from build123d import *

# Parameters (mm, degrees)
F1_DEPTH = 774.7
F2_W     = 304.8
F2_H     = 165.1
F2_R     = 15.875
F2_W_2   = 203.2
F3_DEPTH = 25.4
F4_W     = 88.9
F4_H     = 558.8
F4_R     = 14.2875
F5_DEPTH = 38.1
F6_W     = 12.7
F6_H     = 698.5
F7_DEPTH = 406.4


with BuildPart() as f1:
    # F0 (on Right) → F1 (new body, symmetric)
    with BuildSketch(Plane.YZ):
        with BuildLine():
            Line((-488.95, 12.7), (-488.95, 0))
            Line((-488.95, 0), (-381, 0))
            ThreePointArc((-381, 0), (-358.54936, 9.29936), (-349.25, 31.75))
            Line((-349.25, 31.75), (-349.25, 387.35))
            ThreePointArc((-349.25, 387.35), (-343.670384, 400.820384), (-330.2, 406.4))
            Line((-330.2, 406.4), (0, 406.4))
            Line((0, 406.4), (0, 419.1))
            Line((0, 419.1), (-330.2, 419.1))
            ThreePointArc((-330.2, 419.1), (-352.65064, 409.80064), (-361.95, 387.35))
            Line((-361.95, 387.35), (-361.95, 31.75))
            ThreePointArc((-361.95, 31.75), (-367.529616, 18.279616), (-381, 12.7))
            Line((-381, 12.7), (-488.95, 12.7))
        make_face()
        with BuildLine():
            Line((0, 419.1), (0, 406.4))
            Line((0, 406.4), (330.2, 406.4))
            ThreePointArc((330.2, 406.4), (343.670384, 400.820384), (349.25, 387.35))
            Line((349.25, 387.35), (349.25, 31.75))
            ThreePointArc((349.25, 31.75), (358.54936, 9.29936), (381, 0))
            Line((381, 0), (488.95, 0))
            Line((488.95, 0), (488.95, 12.7))
            Line((488.95, 12.7), (381, 12.7))
            ThreePointArc((381, 12.7), (367.529616, 18.279616), (361.95, 31.75))
            Line((361.95, 31.75), (361.95, 387.35))
            ThreePointArc((361.95, 387.35), (352.65064, 409.80064), (330.2, 419.1))
            Line((330.2, 419.1), (0, 419.1))
        make_face()
    extrude(amount=F1_DEPTH, both=True)

    # F2 (on face) → F3 (join)
    with BuildSketch(Plane.XY.offset(419.1)):
        with Locations((-341.376, 247.65)):
            Rectangle(F2_W, F2_H)
        with Locations((-398.526, 260.35)):
            Circle(F2_R, mode=Mode.SUBTRACT)
        with Locations((255.524, 247.65)):
            Rectangle(F2_W_2, F2_H)
        with Locations((261.874, 260.35)):
            Circle(F2_R, mode=Mode.SUBTRACT)
        with Locations((-341.376, -247.65)):
            Rectangle(F2_W, F2_H)
        with Locations((-398.526, -260.35)):
            Circle(F2_R, mode=Mode.SUBTRACT)
        with Locations((255.524, -247.65)):
            Rectangle(F2_W_2, F2_H)
        with Locations((261.874, -260.35)):
            Circle(F2_R, mode=Mode.SUBTRACT)
    extrude(amount=F3_DEPTH)

    # F4 (on face) → F5 (join, through all)
    with BuildSketch(Plane(origin=(0, 0, 406.4), x_dir=(1, 0, 0), z_dir=(0, 0, -1))):
        with Locations((449.326, 0)):
            Rectangle(F4_W, F4_H)
        with Locations((449.072, -190.5)):
            Circle(F4_R, mode=Mode.SUBTRACT)
        with Locations((449.072, 190.5)):
            Circle(F4_R, mode=Mode.SUBTRACT)
        with Locations((722.122, 0)):
            Rectangle(F4_W, F4_H)
        with Locations((722.376, -190.5)):
            Circle(F4_R, mode=Mode.SUBTRACT)
        with Locations((722.376, 190.5)):
            Circle(F4_R, mode=Mode.SUBTRACT)
    extrude(amount=-F5_DEPTH)

    # F6 (on face) → F7 (join, through all)
    with BuildSketch(Plane(origin=(0, 0, 406.4), x_dir=(1, 0, 0), z_dir=(0, 0, -1))):
        with Locations((-487.426, 0)):
            Rectangle(F6_W, F6_H)
        with Locations((160.274, 0)):
            Rectangle(F6_W, F6_H)
        with Locations((604.774, 0)):
            Rectangle(F6_W, F6_H)
    extrude(amount=F7_DEPTH)


solid = f1.part
Part model, mm, in its own coordinate system. A direction names the side the tool comes from. Give positions to 0.01 mm unless a question says otherwise; leave off trailing zeros. Loops run counter-clockwise (first coordinate to the right, second up) from the corner with the lowest first, then second, coordinate; pieces in that order, holes last. Notation, with made-up numbers: M 25,-30 L 77,-30 A12 ccw 77,-25 Z; hole C -16.75,18.25 d10. An arc over 180 degrees is marked long. Put each result on its own line as item: value. Start each with the question number.
1) Saw through at D-D (x = -27.5). List the corners of the cut face in (y, z), then the cut area to 3 significant figures.
2) Pull direction X, two halves, no side cores. Call faces 6 (the flat face through (774.7, 179, 412)), 7 (the flat face through (449, 191, 419.1)), 8 (the flat face through (386, 349.25, 212)), 9 (the flat face through (11, 436, 12.7)): +X half, -X half, draft (parallel to the pull), parting line (faces both ways), or undercut.
3) 3-axis set-ups, long thin cutter, end or side, ignore diameter. For faces 1 (the flat face through (694, -349.25, 207)), 2 (the cylindrical face through (462.7, 186.21, 431.62)), 3 (the flat face through (11, -434, 12.7)), 4 (the flat face through (-632, -349.25, 207)), 5 (the flat face through (598.424, 5, 206)): which of +Z, -Z, +X, -X, +Y, -Y reach the whole face in a straight line?
4) Flat gauge pins, fed straight in: pin 1 (8 mm diameter, centred on x = 271, z = 169, fed in from -Y); pin 2 (2 mm diameter, centred on y = 296.5, z = 143.5, fed in from -X); pin 3 (12.5 mm diameter, centred on y = -248, z = 432.5, fed in from +X). Where does each tip first touch, or does it go through?
5) Saw through at A-A (z = 240). List the corners of the cut face in (x, y), then the cut area to 3 significant figures.
6) Saw through at B-B (x = -254). List the corners of the cut face in (y, z).
7) Saw through at C-C (y = 25.5). List the corners of the cut face in (x, z), then the cut area to 3 significant figures.
8) Probe probe 1 along X at (y, z) = (190, 424); probe 2 along X at (y, z) = (-193.5, 18); probe 3 along X at (y, z) = (260, 429). List the from-to ranges inside material, lowest first.
Numbers:
1. outline: M -488.95,0 L -381,0 A31.75 ccw -349.25,31.75 L -349.25,387.35 A19.05 cw -330.2,406.4 L 330.2,406.4 A19.05 cw 349.25,387.35 L 349.25,31.75 A31.75 ccw 381,0 L 488.95,0 L 488.95,12.7 L 381,12.7 A19.05 cw 361.95,31.75 L 361.95,387.35 A31.75 ccw 330.2,419.1 L -330.2,419.1 A31.75 ccw -361.95,387.35 L -361.95,31.75 A19.05 cw -381,12.7 L -488.95,12.7 Z
1. area: 22,200 mm^2
2. face 6: +X half
2. face 7: undercut
2. face 8: undercut
2. face 9: draft
3. face 1: -Z, +X
3. face 2: +Z
3. face 3: +Z, +X, -X, -Y
3. face 4: -Z, -X
3. face 5: -Z
4. pin 1: y = -361.95
4. pin 2: x = -493.78
4. pin 3: x = 766.57
5. outline: M -774.7,-361.95 L 774.7,-361.95 L 774.7,-349.25 L 611.12,-349.25 L 611.12,349.25 L 774.7,349.25 L 774.7,361.95 L -774.7,361.95 L -774.7,349.25 L -493.78,349.25 L -493.78,-349.25 L -774.7,-349.25 Z; hole M -481.08,-349.25 L 153.92,-349.25 L 153.92,349.25 L -481.08,349.25 Z; hole M 166.62,-349.25 L 598.42,-349.25 L 598.42,349.25 L 166.62,349.25 Z
5. area: 66,000 mm^2
6. outline: M -488.95,0 L -381,0 A31.75 ccw -349.25,31.75 L -349.25,387.35 A19.05 cw -330.2,406.4 L 330.2,406.4 A19.05 cw 349.25,387.35 L 349.25,31.75 A31.75 ccw 381,0 L 488.95,0 L 488.95,12.7 L 381,12.7 A19.05 cw 361.95,31.75 L 361.95,387.35 A31.75 ccw 330.2,419.1 L 330.2,444.5 L 165.1,444.5 L 165.1,419.1 L -165.1,419.1 L -165.1,444.5 L -330.2,444.5 L -330.2,419.1 A31.75 ccw -361.95,387.35 L -361.95,31.75 A19.05 cw -381,12.7 L -488.95,12.7 Z
7. outline: M -774.7,406.4 L -493.78,406.4 L -493.78,0 L -481.08,0 L -481.08,406.4 L 153.92,406.4 L 153.92,0 L 166.62,0 L 166.62,406.4 L 598.42,406.4 L 598.42,0 L 611.12,0 L 611.12,406.4 L 774.7,406.4 L 774.7,419.1 L 766.57,419.1 L 766.57,444.5 L 677.67,444.5 L 677.67,419.1 L 493.78,419.1 L 493.78,444.5 L 404.88,444.5 L 404.88,419.1 L -774.7,419.1 Z
7. area: 39,700 mm^2
8. probe 1: -493.78 to -188.98, 153.92 to 357.12, 404.88 to 434.79, 463.35 to 493.78, 677.67 to 708.1, 736.65 to 766.57
8. probe 2: -493.78 to -481.08, 153.92 to 166.62, 598.42 to 611.12
8. probe 3: -493.78 to -414.4, -382.65 to -188.98, 153.92 to 246, 277.75 to 357.12, 404.88 to 493.78, 677.67 to 766.57
